from build123d import *

# Parameters (mm, degrees)
F3_DEPTH = 25
F4_R     = 3
F5_DEPTH = 7
F6_R     = 1
F7_DEPTH = 25


# Not quite as in the source:
# - a feature names something its author has since deleted; it is built from what else it names


with BuildPart() as f1:
    # F0 (on Right) → F1 (revolve)
    with BuildSketch(Plane.YZ):
        Polygon((6.6886462844, 0), (16.8847987071, 0), (16.8847987071, 4.5), (11.6886462844, 7.5), (6.6886462844, 7.5), (6.6886462844, 6.5), (11.6886462844, 6.5), (15.1527478995, 4.5), (6.6886462844, 4.5), align=None)
    revolve(axis=Axis((0, 8.4423993535, 0), (0, 1, 0)))

    # F2 (on face) → F3 (cut)
    with BuildSketch(Plane(origin=(0, 16.8847987071, 0), x_dir=(-1, 0, 0), z_dir=(0, 1, 0))):
        with BuildLine():
            ThreePointArc((-7.1139610307, -2.3751965085), (-6.4951905284, -3.75), (-5.6139610307, -4.9732727199))
            Line((-5.6139610307, -4.9732727199), (-3.147114317, -3.5490381057))
            Line((-3.147114317, -3.5490381057), (-3.8971148018, -2.2499991604))
            Line((-3.8971148018, -2.2499991604), (-4.647114317, -0.9509618943))
            Line((-4.647114317, -0.9509618943), (-7.1139610307, -2.3751965085))
        make_face()
        with BuildLine():
            Line((-3.147114317, 3.5490381057), (-5.6139610307, 4.9732727199))
            ThreePointArc((-5.6139610307, 4.9732727199), (-6.4951905284, 3.75), (-7.1139610307, 2.3751965085))
            Line((-7.1139610307, 2.3751965085), (-4.647114317, 0.9509618943))
            Line((-4.647114317, 0.9509618943), (-3.8971148073, 2.2499991508))
            Line((-3.8971148073, 2.2499991508), (-3.147114317, 3.5490381057))
        make_face()
        with BuildLine():
            Line((1.5, 4.5), (1.5, 7.3484692283))
            ThreePointArc((1.5, 7.3484692283), (0, 7.5), (-1.5, 7.3484692283))
            Line((-1.5, 7.3484692283), (-1.5, 4.5))
            Line((-1.5, 4.5), (0, 4.5))
            Line((0, 4.5), (1.5, 4.5))
        make_face()
        with BuildLine():
            Line((4.647114317, 0.9509618943), (7.1139610307, 2.3751965085))
            ThreePointArc((7.1139610307, 2.3751965085), (6.4951905284, 3.75), (5.6139610307, 4.9732727199))
            Line((5.6139610307, 4.9732727199), (3.147114317, 3.5490381057))
            Line((3.147114317, 3.5490381057), (3.8971147984, 2.2499991663))
            Line((3.8971147984, 2.2499991663), (4.647114317, 0.9509618943))
        make_face()
        with BuildLine():
            ThreePointArc((5.6139610307, -4.9732727199), (6.4951905284, -3.75), (7.1139610307, -2.3751965085))
            Line((7.1139610307, -2.3751965085), (4.647114317, -0.9509618943))
            Line((4.647114317, -0.9509618943), (3.8971147929, -2.2499991758))
            Line((3.8971147929, -2.2499991758), (3.147114317, -3.5490381057))
            Line((3.147114317, -3.5490381057), (5.6139610307, -4.9732727199))
        make_face()
        with BuildLine():
            ThreePointArc((-1.5, -7.3484692283), (0, -7.5), (1.5, -7.3484692283))
            Line((1.5, -7.3484692283), (1.5, -4.5))
            Line((1.5, -4.5), (0, -4.5))
            Line((0, -4.5), (-1.5, -4.5))
            Line((-1.5, -4.5), (-1.5, -7.3484692283))
        make_face()
    extrude(amount=-F3_DEPTH, mode=Mode.SUBTRACT)

    # F4 (on face) → F5 (cut)
    with BuildSketch(Plane(origin=(0, 16.8847987071, 0), x_dir=(-1, 0, 0), z_dir=(0, 1, 0))):
        Circle(F4_R)
    extrude(amount=-F5_DEPTH, mode=Mode.SUBTRACT)

    # F6 (on face) → F7 (cut)
    with BuildSketch(Plane(origin=(0, 9.8847987071, 0), x_dir=(-1, 0, 0), z_dir=(0, 1, 0))):
        Circle(F6_R)
    extrude(amount=-F7_DEPTH, mode=Mode.SUBTRACT)


solid = f1.part
Input: part model. Units: mm. Frame: model coordinates. A direction names the side the tool comes from. Coordinates: 2 decimals unless noted, no trailing zeros. Order: outer loops, then holes, each group sorted by start corner. A loop starts at its lowest first (then second) coordinate and runs counter-clockwise, first axis right, second up. Notation, with made-up numbers: M -12,-25.75 L 39,-25.75 A9 cw 39,-14.75 Z; hole C 66,-31 d7. An arc over 180 degrees is marked long. Write item = value, one per line. Start each with the question number.
(1) Pull-direction query (Z, two-part tool) for faces 1 (the flat face through (-1, 6.689, 1)), 2 (the conical face through (3.05, 14.25, -5.19)), 3 (the cylindrical face through (-6.5, 9.2, 0)); classes: released by +Z, released by -Z, zero draft, split by the parting line, or undercut.
(2) Section A-A on y = 8. Output: boundary loops of the cut face in (x, z), and give its area (3 significant figures).
(3) Reachability of faces 4 (the cylindrical face through (6.5, 9.2, 0)), 5 (the flat face through (-4.93, 10.87, 4.58)), 6 (the flat face through (1, 9.885, 1)), 7 (the flat face through (-6.423, 11.237, 1.976)) from +Z, -Z, +X, -X, +Y, -Y: full face, straight path, thin tool, end or side. Return the list, or none.
(4) First-contact query: P1, Ø0.9, axis at y = 12.5, z = -5.5, coming from the +X side; P2, Ø2.5, axis at x = 0.5, y = 15.5, coming from the +Z side; P3, Ø1, axis at y = 14.5, z = 3.5, coming from the +X side. Flat tips, straight axial feed; report the tip coordinate or a pass-through.
(5) Line query: line 1 along Z through (x, y) = (-2.5, 13.25); line 2 along Z through (x, y) = (3.75, 14); line 3 along X through (y, z) = (9.5, 1.5). Output: solid intervals per line, ascending. Write a range as [from, to].
(6) Section C-C on y = 14. Output: boundary loops of the cut face in (x, z).
(7) Section B-B on z = 0. Output: boundary loops of the cut face in (x, y), and give its area (3 significant figures).
(8) Section D-D on x = -4.25. Give the number of separate pieces and of enclosed holes in the cut face, and give its area (3 significant figures).
Result set:
q1.face_1 = zero draft
q1.face_2 = released by -Z
q1.face_3 = undercut
q2.outline = M -7.11,-2.38 L -6.23,-1.86 A6.5 cw -6.23,1.86 L -7.11,2.38 A7.5 ccw Z; M -5.61,-4.97 A7.5 ccw -1.5,-7.35 L -1.5,-6.32 A6.5 cw -4.73,-4.46 Z; M -5.61,4.97 L -4.73,4.46 A6.5 cw -1.5,6.32 L -1.5,7.35 A7.5 ccw Z; C 0,0 d9; M 1.5,-7.35 A7.5 ccw 5.61,-4.97 L 4.73,-4.46 A6.5 cw 1.5,-6.32 Z; M 1.5,6.32 A6.5 cw 4.73,4.46 L 5.61,4.97 A7.5 ccw 1.5,7.35 Z; M 6.23,-1.86 L 7.11,-2.38 A7.5 ccw 7.11,2.38 L 6.23,1.86 A6.5 cw Z; hole C 0,0 d2
q2.area = 86.3 mm²
q3.face_4 = -Y
q3.face_5 = -X, +Y, -Y
q3.face_6 = +Y
q3.face_7 = +Z, +Y, -Y
q4.P1 = 5.02
q4.P2 = 5.53
q4.P3 = 3.93
q5.line_1 = [-6.11, -5.01], [-3.74, -1.66], [1.66, 3.74], [5.01, 6.11]
q5.line_2 = [-4.89, -3.9], [-2.49, 2.49], [3.9, 4.89]
q5.line_3 = [-7.35, -6.32], [-4.24, 4.24], [6.32, 7.35]
q6.outline = M -5.93,-1.69 L -5.03,-1.17 A5.17 cw -5.03,1.17 L -5.93,1.69 A6.17 ccw Z; C 0,0 d9; M -4.43,-4.29 A6.17 ccw -1.5,-5.98 L -1.5,-4.94 A5.17 cw -3.53,-3.77 Z; M -4.43,4.29 L -3.53,3.77 A5.17 cw -1.5,4.94 L -1.5,5.98 A6.17 ccw Z; M 1.5,-5.98 A6.17 ccw 4.43,-4.29 L 3.53,-3.77 A5.17 cw 1.5,-4.94 Z; M 1.5,4.94 A5.17 cw 3.53,3.77 L 4.43,4.29 A6.17 ccw 1.5,5.98 Z; M 5.03,-1.17 L 5.93,-1.69 A6.17 ccw 5.93,1.69 L 5.03,1.17 A5.17 cw Z; hole C 0,0 d6
q7.outline = M -7.5,6.69 L -6.5,6.69 L -6.5,11.69 L -4.5,15.15 L -4.5,6.69 L -1,6.69 L -1,9.88 L -3,9.88 L -3,16.88 L -4.5,16.88 L -7.5,11.69 Z; M 1,6.69 L 4.5,6.69 L 4.5,15.15 L 6.5,11.69 L 6.5,6.69 L 7.5,6.69 L 7.5,11.69 L 4.5,16.88 L 3,16.88 L 3,9.88 L 1,9.88 Z
q7.area = 62.0 mm²
q8.separate_pieces = 3
q8.enclosed_holes = 0
q8.area = 48.1 mm²
